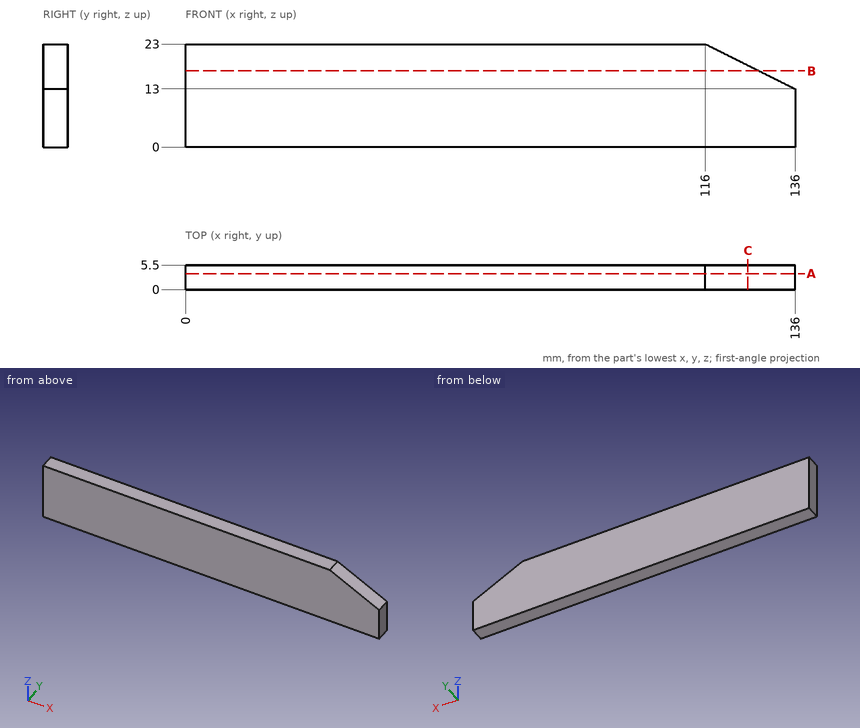
For this review, use the dimensioned drawing (mm, ordinates from the lowest corner) and the shaded views. Round coordinates to 2 decimals unless told otherwise and drop trailing zeros. Write each loop counter-clockwise with the first axis right and the second up, starting at its lowest first coordinate (ties: lowest second). Pieces come first, ordered by that corner, then holes. Notation, with made-up numbers: (44, 16) -> (101, 16) arc R33 ccw to (101, 49) -> close; hole circle Ø7 at (4.25, 32). An arc over 180 degrees is marked (long way). One line per item, written item: value. Start each with the question number.
Q1. Add section A-A (y = 3.6). Give the boundary of the cut face in (x, z), then the cut area to 3 significant figures.
Q2. To check wall thickness, follow probe 1 along X at (y, z) = (4.65, 18); probe 2 along X at (y, z) = (4.15, 20); probe 3 along Z at (x, y) = (123, 4.8). State the ranges of each line that lie inside material, in increasing order.
Q3. Add section C-C (x = 125.5). Give the boundary of the cut face in (y, z), then the cut area to 3 significant figures.
Q4. Add section B-B (z = 17). Give the boundary of the cut face in (x, y), then the cut area to 3 significant figures.
Response:
1. outline: (0, 0) -> (136, 0) -> (136, 13) -> (116, 23) -> (0, 23) -> close
1. area: 3,030 mm^2
2. probe 1: x = 0 to 126
2. probe 2: x = 0 to 122
2. probe 3: z = 0 to 19.5
3. outline: (0, 0) -> (5.5, 0) -> (5.5, 18.25) -> (0, 18.25) -> close
3. area: 100 mm^2
4. outline: (0, 0) -> (128, 0) -> (128, 5.5) -> (0, 5.5) -> close
4. area: 704 mm^2
